Design review of the part shown in the three views and the two pictorial views. Dimensions are in mm from the part's minimum x, y and z. Coordinates: 2 decimals unless noted, no trailing zeros. Write each loop counter-clockwise with the first axis right and the second up, starting at its lowest first coordinate (ties: lowest second). Pieces come first, ordered by that corner, then holes. Notation, with made-up numbers: (12, 63) -> (56, 63) arc R19 ccw to (56, 86) -> close; hole circle Ø11 at (-14, -13.75). An arc over 180 degrees is marked (long way). Write each question's results on one line, items separated by ' | '.
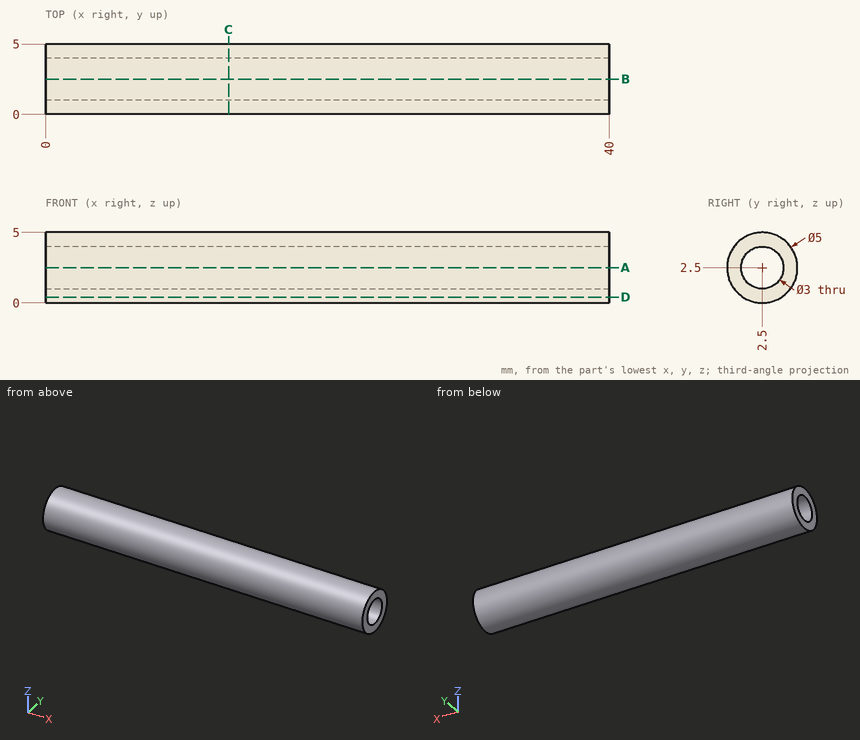
Q1. Add section D-D (z = 0.4). Write out the cut boundary in (x, y).
Solution:
outline: (0, 1.14) -> (40, 1.14) -> (40, 3.86) -> (0, 3.86) -> close
Q2. Add section A-A (z = 2.5). Write out the cut boundary in (x, y), plus the area to 3 significant figures.
Solution:
outline: (0, 0) -> (40, 0) -> (40, 1) -> (0, 1) -> close; (0, 4) -> (40, 4) -> (40, 5) -> (0, 5) -> close | area: 80.0 mm²
Q3. For line 1 (Z direction, x = 15, y = 2.5); line 2 (Z direction, x = 10, y = 3.4), list the stretches that pass through material, from the lowest coordinate up. Write a range as from..to.
Solution:
line 1: 0..1, 4..5 | line 2: 0.17..1.3, 3.7..4.83
Q4. Add section C-C (x = 13). Write out the cut boundary in (y, z), plus the area to 3 significant figures.
Solution:
outline: circle Ø5 at (2.5, 2.5); hole circle Ø3 at (2.5, 2.5) | area: 12.6 mm²
Q5. Clearance check with flat-ended pins moving along their axes: P1, Ø2, axis at x = 23.5, y = 4, coming from the +Z side; P2, Ø2, axis at x = 24.5, z = 4, coming from the -Y side; P3, Ø3, axis at y = 1, z = 2.5, coming from the -X side; P4, Ø1.5, axis at x = 8.5, y = 1.5, coming from the -Z side. State where each tip first meets the part, or that it passes through.
Solution:
P1: z = 4.95 | P2: y = 0.05 | P3: x = 0 | P4: z = 0.01
